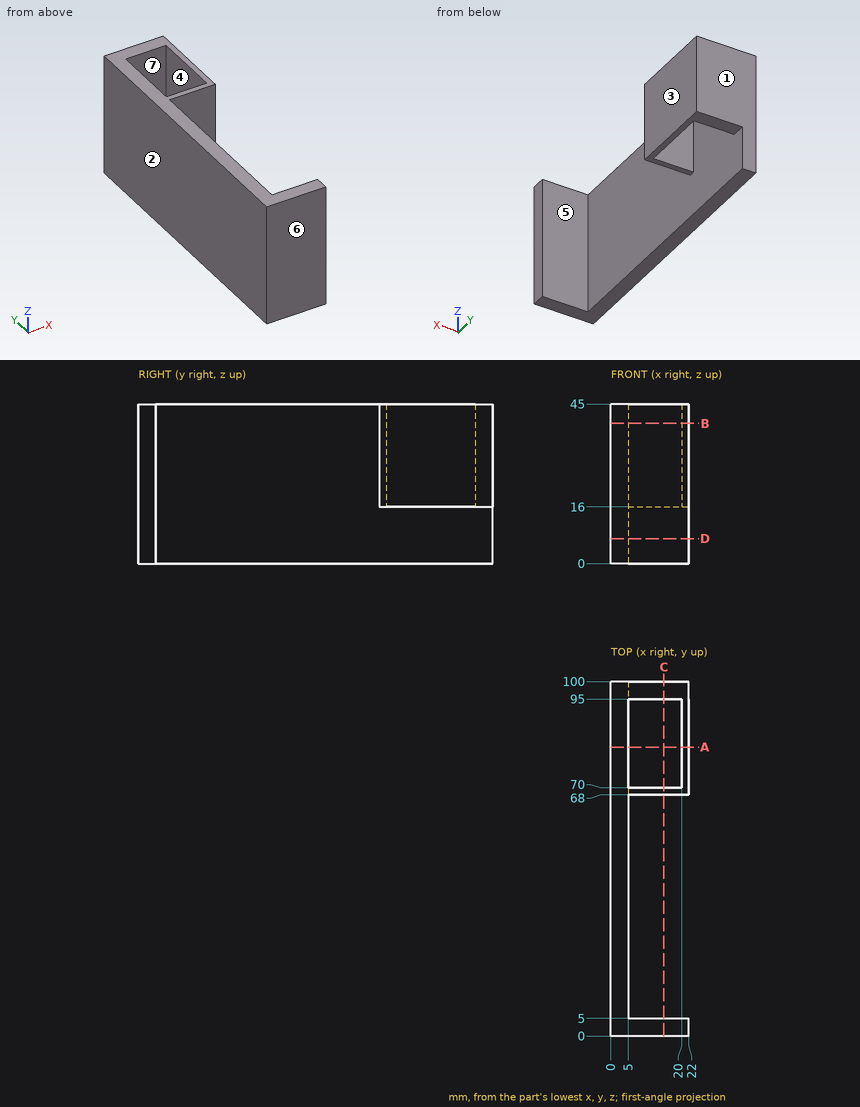
Here's the drawing with two shaded views (mm, measured from the low corner). I have some questions. A direction names the side the tool comes from. Round coordinates to 2 decimals unless told otherwise and drop trailing zeros. Loops run counter-clockwise (first coordinate to the right, second up) from the corner with the lowest first, then second, coordinate; pieces in that order, holes last.
Item 1: Please list where these lines run through material, in increasing order: L1, parallel to Y at x = 9.5, z = 28; L2, parallel to X at y = 85.5, z = 25; L3, parallel to Z at x = 19.75, y = 69.
Item 2: Which directions (+Z, -Z, +X, -X, +Y, -Y) give clear straight access to the entire face, cutting with the end or side of a thin tool? Please do the marked faces 5, 6 and 7.
Item 3: Suppose I cut it at C-C, the plane x = 15. Write out the boundary of the cut face in (y, z), then the cut area to 3 significant figures.
Item 4: Will these pins go through, and if not, where does the flat tip stop? pin 1 Ø6 at (y, z) = (65, 13.5) entering from -X; pin 2 Ø10 at (y, z) = (24.5, 24.5) entering from +X.
Item 5: If we mould it in two halves opening along X, with no side actions, what happens to the marked faces 1, 2, 3 and 4? For each: +X half, -X half, draft (parallel to the pull), parting line (faces both ways), or undercut.
Item 6: Suppose I cut it at B-B, the plane z = 39.5. Write out the boundary of the cut face in (x, y), then the cut area to 3 significant figures.
Item 7: Suppose I cut it at A-A, the plane y = 81.5. Write out the boundary of the cut face in (x, z), then the cut area to 3 significant figures.
Item 8: Suppose I cut it at D-D, the plane z = 7. Write out the boundary of the cut face in (x, y).
Reported:
1. L1: y = 0 to 5, 68 to 70, 95 to 100
1. L2: x = 0 to 5, 20 to 22
1. L3: z = 16 to 45
2. face 5: +Z, -Z, +X
2. face 6: +Z, -Z, +X, -X, -Y
2. face 7: +Z, -Z
3. outline: (0, 0) - (5, 0) - (5, 45) - (0, 45) - close; (68, 16) - (70, 16) - (70, 45) - (68, 45) - close; (95, 16) - (100, 16) - (100, 45) - (95, 45) - close
3. area: 428 mm2
4. pin 1: stops at x = 0
4. pin 2: stops at x = 5
5. face 1: draft
5. face 2: -X half
5. face 3: +X half
5. face 4: undercut
6. outline: (0, 0) - (22, 0) - (22, 5) - (5, 5) - (5, 68) - (22, 68) - (22, 100) - (0, 100) - close; hole (5, 70) - (20, 70) - (20, 95) - (5, 95) - close
6. area: 754 mm2
7. outline: (0, 0) - (5, 0) - (5, 45) - (0, 45) - close; (20, 16) - (22, 16) - (22, 45) - (20, 45) - close
7. area: 283 mm2
8. outline: (0, 0) - (22, 0) - (22, 5) - (5, 5) - (5, 100) - (0, 100) - close
